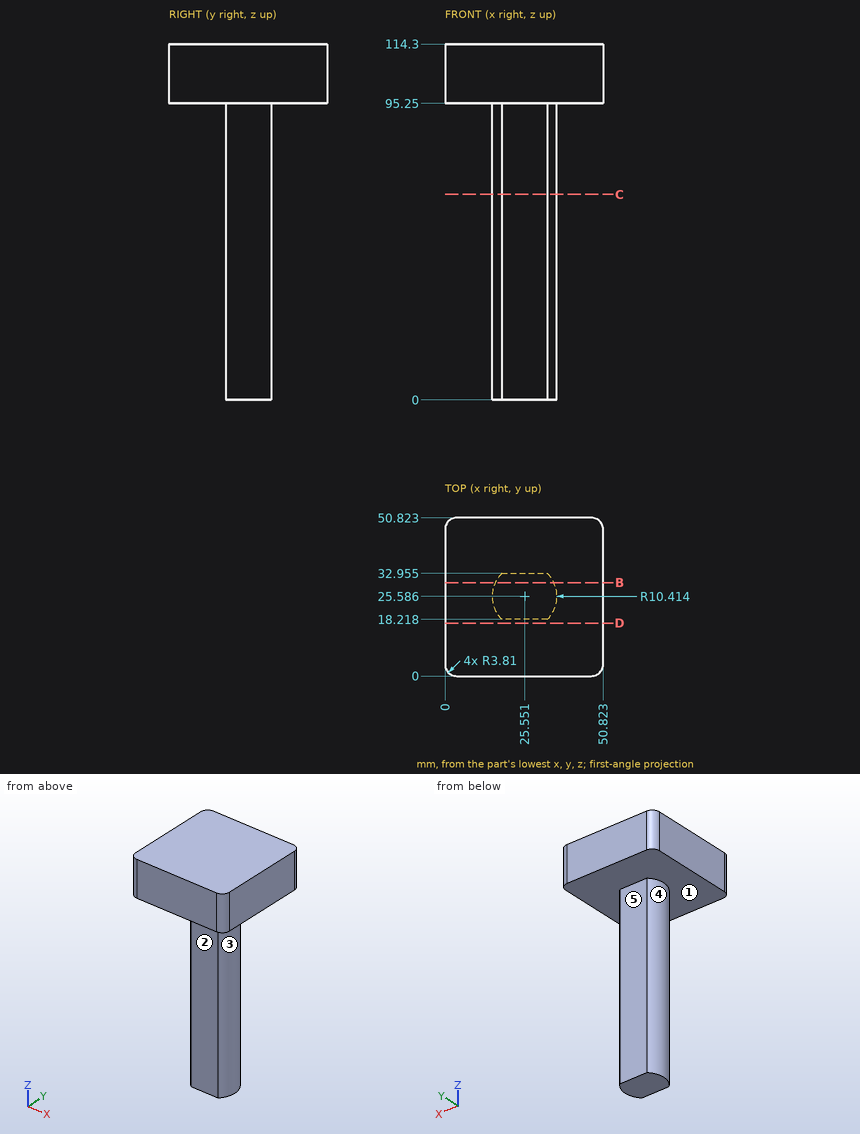
Drawing for the job (mm, zero at the part's lowest x, y, z). A direction names the side the tool comes from. Round coordinates to 2 decimals unless told otherwise and drop trailing zeros. Loops run counter-clockwise (first coordinate to the right, second up) from the corner with the lowest first, then second, coordinate; pieces in that order, holes last.
1. Band-saw the part on B-B, the plane y = 30. List the corners of the cut face in (x, z).
Check values:
outline: (0, 95.25) - (16.12, 95.25) - (16.12, 0) - (34.98, 0) - (34.98, 95.25) - (50.82, 95.25) - (50.82, 114.3) - (0, 114.3) - close
2. Band-saw the part on D-D, the plane y = 17. List the corners of the cut face in (x, z), and give its area (3 significant figures).
Check values:
outline: (0, 95.25) - (50.82, 95.25) - (50.82, 114.3) - (0, 114.3) - close
area: 968 mm2
3. Tool access for the marked faces 1, 2, 3, 4 and 5: list every direction of +Z, -Z, +X, -X, +Y, -Y with a clear straight run to the whole face (end or side of a thin tool).
Check values:
face 1: -Z
face 2: -Z, +X, -X, -Y
face 3: -Z, +X
face 4: -Z, -X
face 5: -Z, +X, -X, +Y
4. Wall check: probe 1 along Z at (x, y) = (48, 47); probe 2 along Y at (x, z) = (28, 65) (1 decimal); probe 3 along Y at (x, z) = (33.5, 51.5) (1 decimal). Give the ranges that are in metal, low to high.
Check values:
probe 1: z = 95.25 to 114.3
probe 2: y = 18.2 to 33
probe 3: y = 18.9 to 32.3
5. Band-saw the part on C-C, the plane z = 66. List the corners of the cut face in (x, y) (1 decimal), and give its area (3 significant figures).
Check values:
outline: (18.2, 18.2) - (32.9, 18.2) arc R10.4 ccw to (32.9, 33) - (18.2, 33) arc R10.4 ccw to start
area: 279 mm2
6. Drop flat-ended pins along their axis: P1, Ø1.5, axis at x = 43, y = 28, coming from the -Z side; P2, Ø16, axis at x = 28.5, z = 24.5, coming from the -Y side; P3, Ø4.5, axis at x = 27.5, z = 41, coming from the +Y side (1 decimal). Give the stop position or say it passes through.
Check values:
P1: stops at z = 95.25
P2: stops at y = 18.22
P3: stops at y = 33
